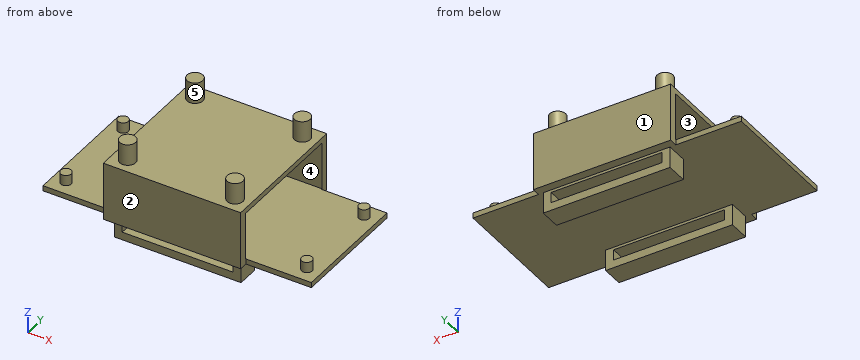
```python
from build123d import *

# Parameters (mm, degrees)
EXTRUDE_1_DEPTH     = 1
SKETCH_3_R          = 1
EXTRUDE_2_DEPTH     = 2
SKETCH_9_W          = 26
SKETCH_9_H          = 1.4
EXTRUDE_4_DEPTH     = 9
SKETCH_10_W         = 26
SKETCH_10_H         = 26
EXTRUDE_5_DEPTH     = 1
SKETCH_11_R         = 1.5
EXTRUDE_6_DEPTH     = 4
SKETCH_6_W          = 24
SKETCH_6_H          = 4
EXTRUDE_7_DEPTH     = 4
SKETCH_12_W         = 21
SKETCH_12_H         = 2
CUT_EXTRUDE_3_DEPTH = 25


with BuildPart() as part:
    # 草图1 → 凸台-拉伸1 (new body)
    with BuildSketch(Plane.XY):
        Polygon((-13, -11.43), (-13, -13), (13, -13), (13, -11.43), (25.4, -11.43), (25.4, 11.43), (13, 11.43), (13, 13), (-13, 13), (-13, 11.43), (-25.4, 11.43), (-25.4, -11.43), align=None)
    extrude(amount=EXTRUDE_1_DEPTH)

    # 草图3 → 凸台-拉伸2 (add)
    with BuildSketch(Plane.XY.offset(1)):
        with Locations(Location((-22.8, -8.63, 0), (0, 0, 180))):
            Circle(SKETCH_3_R)
        with Locations(Location((-22.8, 8.63, 0), (0, 0, 180))):
            Circle(SKETCH_3_R)
        with Locations(Location((22.8, -8.63, 0), (0, 0, 180))):
            Circle(SKETCH_3_R)
        with Locations(Location((22.8, 8.63, 0), (0, 0, 180))):
            Circle(SKETCH_3_R)
    extrude(amount=EXTRUDE_2_DEPTH)

    # 草图9 → 凸台-拉伸4 (add)
    with BuildSketch(Plane.XY.offset(1)):
        with Locations((0, 12.3)):
            Rectangle(SKETCH_9_W, SKETCH_9_H)
        with Locations((0, -12.3)):
            Rectangle(SKETCH_9_W, SKETCH_9_H)
    extrude(amount=EXTRUDE_4_DEPTH)

    # 草图10 → 凸台-拉伸5 (add)
    with BuildSketch(Plane.XY.offset(10)):
        Rectangle(SKETCH_10_W, SKETCH_10_H)
    extrude(amount=EXTRUDE_5_DEPTH)

    # 草图11 → 凸台-拉伸6 (add)
    with BuildSketch(Plane.XY.offset(11)):
        with Locations((-10.16, -10.16)):
            Circle(SKETCH_11_R)
        with Locations(Location((10.16, -10.16, 0), (0, 0, 180))):
            Circle(SKETCH_11_R)
        with Locations((10.16, 10.16)):
            Circle(SKETCH_11_R)
        with Locations(Location((-10.16, 10.16, 0), (0, 0, 180))):
            Circle(SKETCH_11_R)
    extrude(amount=EXTRUDE_6_DEPTH)

    # 草图6 → 凸台-拉伸7 (add)
    with BuildSketch(Plane(origin=(0, 0, 0), x_dir=(-1, 0, 0), z_dir=(0, 0, -1))):
        with Locations((-0.1, 9.43)):
            Rectangle(SKETCH_6_W, SKETCH_6_H)
        with Locations((-0.1, -9.43)):
            Rectangle(SKETCH_6_W, SKETCH_6_H)
    extrude(amount=EXTRUDE_7_DEPTH)

    # 草图12 → 切除-拉伸3 (cut)
    with BuildSketch(Plane(origin=(0, -11.43, 0), x_dir=(-1, 0, 0), z_dir=(0, -1, 0))):
        with Locations((-0.1, 1.5)):
            Rectangle(SKETCH_12_W, SKETCH_12_H)
    extrude(amount=-CUT_EXTRUDE_3_DEPTH, mode=Mode.SUBTRACT)


solid = part.part
```
Here's how the part is built. I have some questions about the finished solid (model axes, mm). Face numbers are marked on the shaded views. A direction names the side the tool comes from. Give positions to 0.01 mm unless a question says otherwise; leave off trailing zeros. Order: outer loops, then holes, each group sorted by start corner. A loop starts at its lowest first (then second) coordinate and runs counter-clockwise, first axis right, second up. Notation, with made-up numbers: (39.25, 52.5) -> (56.25, 52.5) arc R17 cw to (56.25, 62.5) -> close; hole circle Ø8 at (61, 85). An arc over 180 degrees is marked (long way). Use CSV: the item, a comma, the result in double quotes. Start each with the question number.
Item 1: Suppose I cut it at B-B (z = 5.5). List the corners of the cut face in (x, y) for me, and give its area (3 significant figures).
Item 2: If I drill on probe 1 along Z at (x, y) = (-1, 8.5); probe 2 along Z at (x, y) = (-12, 2); probe 3 along Y at (x, z) = (4, 1.75), over which ranges is the centre line in solid material (lowest first)? Write a range as [from, to].
Item 3: Thinking about a two-plate mould opening in Y: for the marked faces 1, 2 and 3, which applies, pulls with the +Y half, pulls with the -Y half, needs draft (parallel to the pull), parting line crosses it, or undercut?
Item 4: I'm going to push flat-ended pins straight in: P1, Ø8, axis at x = 10.5, y = -2, coming from the -Z side; P2, Ø1.2, axis at x = 2.5, y = 8.5, coming from the +Z side; P3, Ø0.6, axis at x = 22.5, y = -8, coming from the +Z side. Where does each tip first touch, or does it pass through?
Item 5: Suppose I cut it at C-C (x = -2). List the corners of the cut face in (y, z) for me.
Item 6: Suppose I cut it at A-A (y = 10.16). List the corners of the cut face in (x, z) for me.
Item 7: On a 3-axis mill with a long thin cutter (end or side, diameter ignored), from which of +Z, -Z, +X, -X, +Y, -Y can I reach the whole of each face in a straight line? I mean the marked faces 4 and 5. Say none if no direction works.
Item 8: Suppose I cut it at D-D (y = 4.25). List the corners of the cut face in (x, z) for me.
Answer block:
1,outline,"(-13, -13) -> (13, -13) -> (13, -11.6) -> (-13, -11.6) -> close; (-13, 11.6) -> (13, 11.6) -> (13, 13) -> (-13, 13) -> close"
1,area,"72.8 mm^2"
2,probe 1,"z = [-4, -2.5], [-0.5, 1], [10, 11]"
2,probe 2,"z = [0, 1], [10, 11]"
2,probe 3,"y = [-13, -11.6], [11.6, 13]"
3,face 1,"pulls with the +Y half"
3,face 2,"pulls with the -Y half"
3,face 3,"undercut"
4,P1,"stops at z = 0"
4,P2,"stops at z = 11"
4,P3,"stops at z = 3"
5,outline,"(-13, 0) -> (-11.43, 0) -> (-11.43, -0.5) -> (-7.43, -0.5) -> (-7.43, 0) -> (7.43, 0) -> (7.43, -0.5) -> (11.43, -0.5) -> (11.43, 0) -> (13, 0) -> (13, 11) -> (-13, 11) -> close; (-11.43, -4) -> (-7.43, -4) -> (-7.43, -2.5) -> (-11.43, -2.5) -> close; (7.43, -4) -> (11.43, -4) -> (11.43, -2.5) -> (7.43, -2.5) -> close; hole (-11.6, 1) -> (11.6, 1) -> (11.6, 10) -> (-11.6, 10) -> close"
6,outline,"(-25.4, 0) -> (-11.9, 0) -> (-11.9, -4) -> (12.1, -4) -> (12.1, 0) -> (25.4, 0) -> (25.4, 1) -> (-25.4, 1) -> close; (-13, 10) -> (13, 10) -> (13, 11) -> (11.66, 11) -> (11.66, 15) -> (8.66, 15) -> (8.66, 11) -> (-8.66, 11) -> (-8.66, 15) -> (-11.66, 15) -> (-11.66, 11) -> (-13, 11) -> close; hole (-10.4, -2.5) -> (10.6, -2.5) -> (10.6, -0.5) -> (-10.4, -0.5) -> close"
7,face 4,"+X, -X"
7,face 5,"+Z"
8,outline,"(-25.4, 0) -> (25.4, 0) -> (25.4, 1) -> (-25.4, 1) -> close; (-13, 10) -> (13, 10) -> (13, 11) -> (-13, 11) -> close"
